from build123d import *

# Parameters (mm, degrees)
EXTRUDE_1_DEPTH = 2400


with BuildPart() as part:
    # Эскиз1 → Бобышка-Вытянуть1 (new body)
    with BuildSketch(Plane(origin=(0, 0, 0), x_dir=(1, 0, 0), z_dir=(0, 1, 0))):
        with BuildLine():
            Line((20, 35.1), (20, 40))
            Line((20, 40), (-20, 40))
            Line((-20, 40), (-20, -40))
            Line((-20, -40), (20, -40))
            Line((20, -40), (20, -35.1))
            ThreePointArc((20, -35.1), (19.267766953, -33.332233047), (17.5, -32.6))
            Line((17.5, -32.6), (-8, -32.6))
            ThreePointArc((-8, -32.6), (-13.303300859, -30.403300859), (-15.5, -25.1))
            Line((-15.5, -25.1), (-15.5, 25.1))
            ThreePointArc((-15.5, 25.1), (-13.303300859, 30.403300859), (-8, 32.6))
            Line((-8, 32.6), (17.5, 32.6))
            ThreePointArc((17.5, 32.6), (19.267766953, 33.332233047), (20, 35.1))
        make_face()
    extrude(amount=EXTRUDE_1_DEPTH)


solid = part.part
Build history of the part. All positions in model axes, mm. Give positions to 0.01 mm unless a question says otherwise; leave off trailing zeros. Order: outer loops, then holes, each group sorted by start corner. A loop starts at its lowest first (then second) coordinate and runs counter-clockwise, first axis right, second up. Notation, with made-up numbers: M 17.25,12 L 46.25,12 A28 ccw 46.25,38 Z; hole C -31.5,42.5 d10. An arc over 180 degrees is marked long. Put each result on its own line as item: value.
Item 1: Slice it at A-A, the plane y = 1467.5. Write the cut outline in (x, z).
From the geometry:
outline: M -20,-40 L 20,-40 L 20,-35.1 A2.5 ccw 17.5,-32.6 L -8,-32.6 A7.5 cw -15.5,-25.1 L -15.5,25.1 A7.5 cw -8,32.6 L 17.5,32.6 A2.5 ccw 20,35.1 L 20,40 L -20,40 Z
Item 2: Probe line 1 (Z direction, x = 14, y = 556); line 2 (X direction, y = 1727.5, z = 7); line 3 (Z direction, x = 18, y = 608.5). List the from-to ranges inside material, lowest first. Write a range as [from, to].
From the geometry:
line 1: z = [-40, -32.6], [32.6, 40]
line 2: x = [-20, -15.5]
line 3: z = [-40, -32.65], [32.65, 40]
Item 3: Two-plate mould, pull along Z, no slides. Class faces 1 (the flat face through (-15.5, 1183, 0)), 2 (the flat face through (0, 1183, -40)), 3 (the flat face through (-20, 1183, -1)): +Z half, -Z half, draft (parallel to the pull), parting line (faces both ways), or undercut.
From the geometry:
face 1: undercut
face 2: -Z half
face 3: draft
Item 4: Flat gauge pins, fed straight in: pin 1 Ø4 at (y, z) = (1075.5, 25) entering from +X; pin 2 Ø2 at (y, z) = (668.5, 7) entering from +X; pin 3 Ø10 at (y, z) = (464, 23.5) entering from +X. Where does each tip first touch, or does it go through?
From the geometry:
pin 1: stops at x = -15.26
pin 2: stops at x = -15.5
pin 3: stops at x = -14.69
Item 5: Slice it at B-B, the plane z = 8. Write the cut outline in (x, y).
From the geometry:
outline: M -20,0 L -15.5,0 L -15.5,2400 L -20,2400 Z
